Can you work these out from the model? Positions are in its coordinate system, mm. Face numbers are marked on the shaded views. A direction names the side the tool comes from. Coordinates: 2 decimals unless noted, no trailing zeros. Loops run counter-clockwise (first coordinate to the right, second up) from the corner with the lowest first, then second, coordinate; pieces in that order, holes last. Notation, with made-up numbers: M 4,89 L 26,89 A14 cw 26,104 Z; hole C -29,79.25 d11. An arc over 180 degrees is marked long. Return JSON: item names as keys, results as strings. Group by question number.
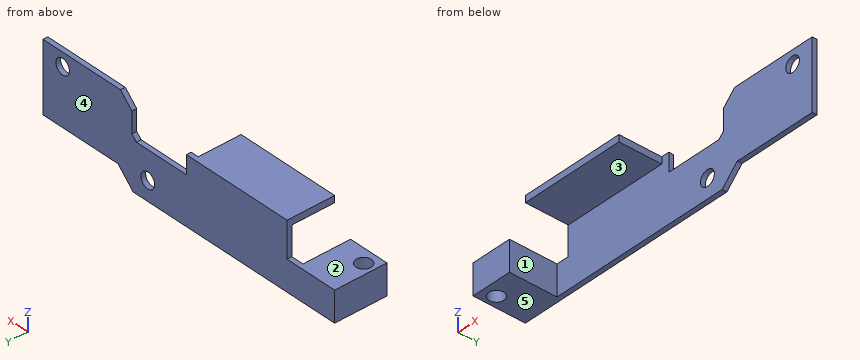
```python
from build123d import *

# Parameters (mm, degrees)
SKETCH_1_R          = 1.632566579
SKETCH_1_R_2        = 1.6
EXTRUDE_1_DEPTH     = 1
SKETCH_2_W          = 21.996438878
SKETCH_2_H          = 1.4
EXTRUDE_2_DEPTH     = 9
SKETCH_3_W          = 9.861847607
SKETCH_3_H          = 7.366382786
EXTRUDE_3_DEPTH     = 10
CUT_EXTRUDE_1_REACH = 9.366
SKETCH_5_R          = 1.6
CUT_EXTRUDE_2_REACH = 13


with BuildPart() as part:
    # 草图1 → 凸台-拉伸1 (new body)
    with BuildSketch(Plane(origin=(0, 0, 0), x_dir=(1, 0, 0), z_dir=(0, 1, 0))):
        Polygon((-59.259088641, 5), (-10.592885375, 5), (-7.033226841, 1.452276921), (10.592885375, 1.452276921), (10.592885375, -5), (10.592885375, -13.105286597), (-7.648958362, -13.105286597), (-10.311746214, -10.442498745), (-10.311746214, -6.049690331), (-11.364057651, -4.997378894), (-11.364090146, -5), (-23.120004307, -5), (-23.120004307, -8.866382786), (-46.772006656, -8.866382786), (-46.772006656, -2.366382786), (-59.259088641, -2.366382786), (-59.259088641, 0), align=None)
        with Locations((-14.039400366, 0.94270398)):
            Circle(SKETCH_1_R, mode=Mode.SUBTRACT)
        with Locations((5.968790226, -10.300345076)):
            Circle(SKETCH_1_R_2, mode=Mode.SUBTRACT)
    extrude(amount=EXTRUDE_1_DEPTH)

    # 草图2 → 凸台-拉伸2 (add)
    with BuildSketch(Plane.XZ):
        with Locations((-35.773787217, 8.166382786)):
            Rectangle(SKETCH_2_W, SKETCH_2_H)
    extrude(amount=EXTRUDE_2_DEPTH)

    # 草图3 → 凸台-拉伸3 (add)
    with BuildSketch(Plane.XZ):
        with Locations((-54.328164838, -1.316808607)):
            Rectangle(SKETCH_3_W, SKETCH_3_H)
    extrude(amount=EXTRUDE_3_DEPTH)

    # 草图5 → 切除-拉伸1 (cut, up to next)
    with BuildSketch(Plane.XY.offset(2.366382786), mode=Mode.PRIVATE) as cut_extrude_1_sk1:
        with Locations((-55.594883285, -7.2)):
            Circle(SKETCH_5_R)
    cut_extrude_1_tool1 = extrude(cut_extrude_1_sk1.sketch, amount=-CUT_EXTRUDE_1_REACH, mode=Mode.PRIVATE) & part.part
    add(cut_extrude_1_tool1.solids().sort_by_distance((-55.594883, -7.2, 2.366383))[0], mode=Mode.SUBTRACT)

    # 草图6 → 切除-拉伸2 (cut, up to next)
    with BuildSketch(Plane(origin=(0, 1, 0), x_dir=(1, 0, 0), z_dir=(0, 1, 0)), mode=Mode.PRIVATE) as cut_extrude_2_sk1:
        Polygon((-59.259088641, 5), (-57.959088641, 5), (-57.959088641, -1.366382786), (-46.772006656, -1.366382786), (-46.772006656, -2.366382786), (-57.959088641, -2.366382786), (-59.259088641, -2.366382786), align=None)
    cut_extrude_2_tool1 = extrude(cut_extrude_2_sk1.sketch, amount=-CUT_EXTRUDE_2_REACH, mode=Mode.PRIVATE) & part.part
    add(cut_extrude_2_tool1.solids().sort_by_distance((-58.609089, 1, -4.85502))[0], mode=Mode.SUBTRACT)


solid = part.part
```
1) If I drill on line 1 (Y direction, x = -30, z = 4.5); line 2 (Z direction, x = -28, y = -8.5); line 3 (Z direction, x = -53, y = -3.75), over which ranges is the centre line in solid material (lowest first)? Write a range as from..to.
2) Suppose I cut it at A-A, the plane y = -7.2. List the corners of the cut face in (x, z) for me.
3) Suppose I cut it at B-B, the plane y = -4.25. List the corners of the cut face in (x, z) for me.
4) For the marked faces 1, 2, 3, 4 and 5, which set-ups out of +Z, -Z, +X, -X, +Y, -Y let a thin tool reach every point of the face, with its end or its side?
5) Suppose I cut it at D-D, the plane x = -32. List the corners of the cut face in (y, z) for me.
6) For pin 1 (1.1 mm diameter, centred on x = -2.5, y = 0.5, fed in from -Z); pin 2 (0.7 mm diameter, centred on y = -4, z = 8.5, fed in from +X); pin 3 (3 mm diameter, centred on y = -5.5, z = -2.5, fed in from +X), each with a flat end and sliding along its axis, tell me the tip position at first contact or that it passes through.
7) Suppose I cut it at C-C, the plane z = -4. List the corners of the cut face in (x, y) for me, then the cut area to 3 significant figures.
Returned:
{
 "1": {"line 1": "y = 0..1", "line 2": "z = 7.47..8.87", "line 3": "z = -5..1.37"},
 "2": {"outline": "M -57.96,-5 L -57.19,-5 L -57.19,1.37 L -57.96,1.37 Z; M -53.99,-5 L -49.4,-5 L -49.4,1.37 L -53.99,1.37 Z; M -46.77,7.47 L -24.78,7.47 L -24.78,8.87 L -46.77,8.87 Z"},
 "3": {"outline": "M -57.96,-5 L -49.4,-5 L -49.4,1.37 L -57.96,1.37 Z; M -46.77,7.47 L -24.78,7.47 L -24.78,8.87 L -46.77,8.87 Z"},
 "4": {"face 1": "+Z, -Z, +X, -Y", "face 2": "+Z, -X, +Y, -Y", "face 3": "-Z, +X, -X, -Y", "face 4": "+Z, -Z, +X, -X, +Y", "face 5": "-Z, +X, -X, +Y, -Y"},
 "5": {"outline": "M -9,7.47 L 0,7.47 L 0,-5 L 1,-5 L 1,8.87 L -9,8.87 Z"},
 "6": {"pin 1": "stops at z = -1.45", "pin 2": "stops at x = -24.78", "pin 3": "stops at x = -49.4"},
 "7": {"outline": "M -57.96,-10 L -49.4,-10 L -49.4,0 L -9.59,0 L -9.59,1 L -57.96,1 Z; hole C -55.59,-7.2 d3.2", "area": "126 mm²"}
}
